Verification items for the finished model (mm, model axes). Give positions to 0.01 mm unless a question says otherwise; leave off trailing zeros. Write item = value, one per line.
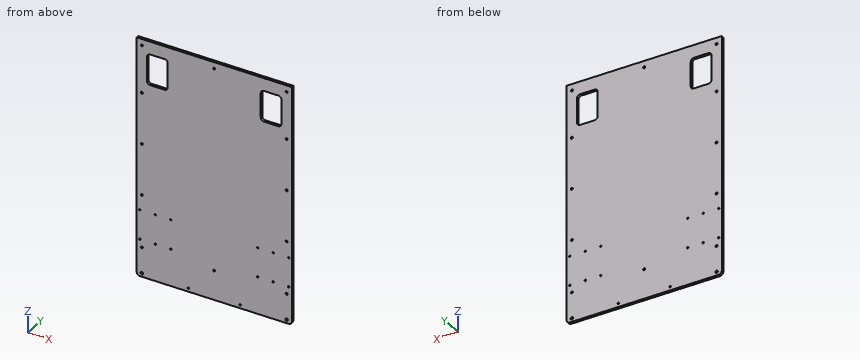
from build123d import *

# Parameters (mm, degrees)
SKETCH1_R           = 2
SKETCH1_R_2         = 1.5
SKETCH1_R_3         = 2.5
SKETCH1_W           = 40
SKETCH1_H           = 60
BOSS_EXTRUDE1_DEPTH = 5
FILLET1_R           = 6


with BuildPart() as part:
    # Sketch1 → Boss-Extrude1 (new body)
    with BuildSketch(Plane(origin=(0, 0, 0), x_dir=(1, 0, 0), z_dir=(0, 1, 0))):
        Polygon((-150, -210), (150, -210), (150, 210), (150, 255), (-150, 255), (-150, 210), align=None)
        with Locations(Location((0, -197.5, 0), (0, 0, 270))):
            Circle(SKETCH1_R, mode=Mode.SUBTRACT)
        with Locations(Location((-140, -197.5, 0), (0, 0, 270))):
            Circle(SKETCH1_R, mode=Mode.SUBTRACT)
        with Locations(Location((-140, 197.5, 0), (0, 0, 270))):
            Circle(SKETCH1_R, mode=Mode.SUBTRACT)
        with Locations(Location((0, 197.5, 0), (0, 0, 270))):
            Circle(SKETCH1_R, mode=Mode.SUBTRACT)
        with Locations(Location((-140, -5, 0), (0, 0, 270))):
            Circle(SKETCH1_R, mode=Mode.SUBTRACT)
        with Locations(Location((-140, 95, 0), (0, 0, 270))):
            Circle(SKETCH1_R, mode=Mode.SUBTRACT)
        with Locations(Location((140, 197.5, 0), (0, 0, 270))):
            Circle(SKETCH1_R, mode=Mode.SUBTRACT)
        with Locations(Location((140, -197.5, 0), (0, 0, 270))):
            Circle(SKETCH1_R, mode=Mode.SUBTRACT)
        with Locations(Location((-114, 182.625, 0), (0, 0, 270))):
            Circle(SKETCH1_R_2, mode=Mode.SUBTRACT)
        with Locations(Location((-144, 182.625, 0), (0, 0, 270))):
            Circle(SKETCH1_R_2, mode=Mode.SUBTRACT)
        with Locations(Location((-84, 182.625, 0), (0, 0, 270))):
            Circle(SKETCH1_R_2, mode=Mode.SUBTRACT)
        with Locations(Location((-84, 125.375, 0), (0, 0, 270))):
            Circle(SKETCH1_R_2, mode=Mode.SUBTRACT)
        with Locations(Location((-114, 125.375, 0), (0, 0, 270))):
            Circle(SKETCH1_R_2, mode=Mode.SUBTRACT)
        with Locations(Location((-144, 125.375, 0), (0, 0, 270))):
            Circle(SKETCH1_R_2, mode=Mode.SUBTRACT)
        with Locations(Location((-140, -105, 0), (0, 0, 270))):
            Circle(SKETCH1_R, mode=Mode.SUBTRACT)
        with Locations(Location((-140, 248, 0), (0, 0, 270))):
            Circle(SKETCH1_R_3, mode=Mode.SUBTRACT)
        with Locations(Location((-50, 248, 0), (0, 0, 270))):
            Circle(SKETCH1_R_2, mode=Mode.SUBTRACT)
        with Locations(Location((140, -105, 0), (0, 0, 270))):
            Circle(SKETCH1_R, mode=Mode.SUBTRACT)
        with Locations(Location((140, 95, 0), (0, 0, 270))):
            Circle(SKETCH1_R, mode=Mode.SUBTRACT)
        with Locations(Location((140, -5, 0), (0, 0, 270))):
            Circle(SKETCH1_R, mode=Mode.SUBTRACT)
        with Locations(Location((144, 125.375, 0), (0, 0, 270))):
            Circle(SKETCH1_R_2, mode=Mode.SUBTRACT)
        with Locations(Location((114, 125.375, 0), (0, 0, 270))):
            Circle(SKETCH1_R_2, mode=Mode.SUBTRACT)
        with Locations(Location((84, 125.375, 0), (0, 0, 270))):
            Circle(SKETCH1_R_2, mode=Mode.SUBTRACT)
        with Locations(Location((84, 182.625, 0), (0, 0, 270))):
            Circle(SKETCH1_R_2, mode=Mode.SUBTRACT)
        with Locations(Location((144, 182.625, 0), (0, 0, 270))):
            Circle(SKETCH1_R_2, mode=Mode.SUBTRACT)
        with Locations(Location((114, 182.625, 0), (0, 0, 270))):
            Circle(SKETCH1_R_2, mode=Mode.SUBTRACT)
        with Locations(Location((50, 248, 0), (0, 0, 270))):
            Circle(SKETCH1_R_2, mode=Mode.SUBTRACT)
        with Locations(Location((140, 248, 0), (0, 0, 270))):
            Circle(SKETCH1_R_3, mode=Mode.SUBTRACT)
        with Locations((-110, -155)):
            Rectangle(SKETCH1_W, SKETCH1_H, mode=Mode.SUBTRACT)
        with Locations((110, -155)):
            Rectangle(SKETCH1_W, SKETCH1_H, mode=Mode.SUBTRACT)
    extrude(amount=BOSS_EXTRUDE1_DEPTH)

    # Fillet1
    fillet1_edges = [part.edges().sort_by_distance(p)[0] for p in [
        (130, 2.5, 185),
        (130, 2.5, 125),
        (90, 2.5, 125),
        (90, 2.5, 185),
        (-90, 2.5, 125),
        (-130, 2.5, 125),
        (-130, 2.5, 185),
        (-90, 2.5, 185),
        (-150, 2.5, -255),
        (150, 2.5, -255),
    ]]
    fillet(fillet1_edges, radius=FILLET1_R)


solid = part.part
Item 1: Go/stop test with a flat-tipped pin: P1, Ø3, axis at x = 140, z = -197.5, coming from the +Y side. Record where the tip stops, or that it passes through.
Response values:
P1 = through
Item 2: Material ranges on line 1 (Z direction, x = -84, y = 3.9) (3 decimals); line 2 (X direction, y = 3.2, z = -248); line 3 (Z direction, x = -114, y = 4.45) (3 decimals), recorded low to high.
Response values:
line_1 = -255 to -184.125, -181.125 to -126.875, -123.875 to 210
line_2 = -150 to -142.5, -137.5 to -51.5, -48.5 to 48.5, 51.5 to 137.5, 142.5 to 150
line_3 = -255 to -184.125, -181.125 to -126.875, -123.875 to 125, 185 to 210
Item 3: Sectioned sample at A-A on y = 1.5. Give the number of separate pieces and of enclosed holes in the cut face, then the cut area to 3 significant figures.
Response values:
separate_pieces = 1
enclosed_holes = 30
area = 134,000 mm^2
